```python
from build123d import *

# Parameters (mm, degrees)
BOSS_EXTRUDE1_DEPTH = 72
BOSS_EXTRUDE4_DEPTH = 6
SKETCH5_3_R         = 8.173204637
CUT_EXTRUDE1_DEPTH  = 6
BOSS_EXTRUDE6_START = 5
SKETCH7_R           = 15
BOSS_EXTRUDE6_DEPTH = 5
CUT_EXTRUDE3_START  = 5
SKETCH5_6_R         = 8.173204637
CUT_EXTRUDE3_DEPTH  = 5
RIB6_REACH          = 87.013
SKETCH18_WALL_W     = 218.674083686
SKETCH18_WALL_H     = 10
SKETCH20_R          = 6
CUT_EXTRUDE5_DEPTH  = 99.565967758
FILLET12_R          = 12


with BuildPart() as part:
    # Sketch2 → Boss-Extrude1 (new body)
    with BuildSketch(Plane(origin=(0, 0, 0), x_dir=(0, 0, -1), z_dir=(1, 0, 0))):
        Polygon((-17.5, 0), (-17.5, 6), (-12.5, 6), (-12.5, 10), (17.5, 10), (17.5, 0), align=None)
    extrude(amount=BOSS_EXTRUDE1_DEPTH)

    # Sketch5 → Boss-Extrude4 (add)
    with BuildSketch(Plane.XY.offset(12.5)):
        with BuildLine():
            Line((21, 60), (21, 20.340753373))
            ThreePointArc((21, 20.340753373), (17.971263459, 13.028736541), (10.659246627, 10))
            Line((10.659246627, 10), (61.340753373, 10))
            ThreePointArc((61.340753373, 10), (53.857333501, 15.45146146), (51, 24.258030049))
            Line((51, 24.258030049), (51, 60))
            ThreePointArc((51, 60), (36, 75), (21, 60))
        make_face()
    extrude(amount=-BOSS_EXTRUDE4_DEPTH)

    # Sketch5_3 → Cut-Extrude1 (cut)
    with BuildSketch(Plane.XY.offset(12.5)):
        with Locations((36, 60)):
            Circle(SKETCH5_3_R)
    extrude(amount=-CUT_EXTRUDE1_DEPTH, mode=Mode.SUBTRACT)

    # Sketch7 → Boss-Extrude6 (add)
    with BuildSketch(Plane.XY.offset(12.5).offset(BOSS_EXTRUDE6_START)):
        with Locations((36, 60)):
            Circle(SKETCH7_R)
    extrude(amount=-BOSS_EXTRUDE6_DEPTH)

    # Sketch5_6 → Cut-Extrude3 (cut)
    with BuildSketch(Plane.XY.offset(12.5).offset(CUT_EXTRUDE3_START)):
        with Locations((36, 60)):
            Circle(SKETCH5_6_R)
    extrude(amount=-CUT_EXTRUDE3_DEPTH, mode=Mode.SUBTRACT)

    # Sketch18 wall → Rib6 (add, up to next)
    with BuildSketch(Plane(origin=(36, 30, -5.5), x_dir=(0, -0.857492925713, -0.514495755428), z_dir=(0, 0.514495755428, -0.857492925713)), mode=Mode.PRIVATE) as rib6_sk1:
        Rectangle(SKETCH18_WALL_W, SKETCH18_WALL_H)
    rib6_tool1 = extrude(rib6_sk1.sketch, amount=-RIB6_REACH, mode=Mode.PRIVATE) - part.part
    add(rib6_tool1.solids().sort_by_distance((36, 30, -5.5))[0])

    # Sketch20 → Cut-Extrude5 (cut, through all)
    with BuildSketch(Plane(origin=(0, 10, 0), x_dir=(1, 0, 0), z_dir=(0, 1, 0))):
        with Locations(Location((12, 5.5, 0), (0, 0, 270))):
            Circle(SKETCH20_R)
        with Locations(Location((60, 5.5, 0), (0, 0, 270))):
            Circle(SKETCH20_R)
    extrude(amount=-CUT_EXTRUDE5_DEPTH, mode=Mode.SUBTRACT)

    # Fillet12
    fillet12_edges = [part.edges().sort_by_distance(p)[0] for p in [
        (0, 5, -17.5),
        (72, 5, -17.5),
    ]]
    fillet(fillet12_edges, radius=FILLET12_R)


solid = part.part
```
Part model, mm, in its own coordinate system. A direction names the side the tool comes from. Round coordinates to 2 decimals unless told otherwise and drop trailing zeros. Write each loop counter-clockwise with the first axis right and the second up, starting at its lowest first coordinate (ties: lowest second). Pieces come first, ordered by that corner, then holes. Notation, with made-up numbers: M -5,59 L 32,59 A11 ccw 32,75 Z; hole C 84.5,8.5 d7. An arc over 180 degrees is marked long. Answer as CSV lines item,"result". Start each with the question number.
1) Band-saw the part on B-B (z = 9). List the corners of the cut face in (x, y), then the cut area to 3 significant figures.
2) Mould opens along Z. For faces 4 (the face through (18.05, 13.11, 9.54)), 5 (the face through (6.143, 5.07, -6.801)), 6 (the face through (41.3, 35.7, 6.5)) say: +Z half, -Z half, draft (parallel to the pull), parting line (faces both ways), or undercut.
3) Band-saw the part on C-C (y = 26). List the corners of the cut face in (x, z).
4) Drop flat-ended pins along their axis: pin 1 (4 mm diameter, centred on y = 38, z = 6.5, fed in from +X); pin 2 (7 mm diameter, centred on x = 60, z = -5.5, fed in from -Y); pin 3 (1.5 mm diameter, centred on y = 22, z = 4.5, fed in from +X); pin 4 (12 mm diameter, centred on y = 22.5, z = -4.5, fed in from -X). Give the stop position or say it passes through.
5) Which spindle directions (+Z, -Z, +X, -X, +Y, -Y) get a long thin tool onto all of the face, cutting with end or side? Do faces 1 (the face through (34.047, 74.872, 13.299)), 2 (the face through (21, 40, 10)), 3 (the face through (19, 10, -2)). Say none if no direction does.
6) Drill centre lines: L1, parallel to X at y = 7, z = -5.5; L2, parallel to Y at x = 36, z = 15; L3, parallel to Z at x = 22, y = 62. Where is each one in solid material? Low to high.
7) Band-saw the part on A-A (x = 36). List the corners of the cut face in (y, z), then the cut area to 3 significant figures.
8) Band-saw the part on D-D (z = -6.5). List the corners of the cut face in (x, y).
Worked out:
1,outline,"M 0,0 L 72,0 L 72,10 L 61.34,10 A15 cw 51,24.26 L 51,60 A15 ccw 21,60 L 21,20.34 A10.34 cw 10.66,10 L 0,10 Z; hole C 36,60 d16.35"
1,area,"2,430 mm²"
2,face 4,"draft"
2,face 5,"undercut"
2,face 6,"-Z half"
3,outline,"M 21,6.5 L 31,6.5 L 31,-7.9 L 41,-7.9 L 41,6.5 L 51,6.5 L 51,12.5 L 21,12.5 Z"
4,pin 1,"x = 51"
4,pin 2,"through"
4,pin 3,"x = 41"
4,pin 4,"x = 31"
5,face 1,"+Z"
5,face 2,"+Z, -Z, -X, +Y"
5,face 3,"-Z, -X, +Y"
6,L1,"0 to 6, 18 to 54, 66 to 72"
6,L2,"0 to 6, 45 to 51.83, 68.17 to 75"
6,L3,"6.5 to 17.5"
7,outline,"M 0,-17.5 L 10,-17.5 L 50,6.5 L 51.83,6.5 L 51.83,17.5 L 45,17.5 L 45,12.5 L 6,12.5 L 6,17.5 L 0,17.5 Z; M 68.17,6.5 L 75,6.5 L 75,17.5 L 68.17,17.5 Z"
7,area,"1,170 mm²"
8,outline,"M 0.04,0 L 6.08,0 L 6.08,10 L 0.04,10 Z; M 17.92,0 L 54.08,0 L 54.08,10 L 41,10 L 41,28.33 L 31,28.33 L 31,10 L 17.92,10 Z; M 65.92,0 L 71.96,0 L 71.96,10 L 65.92,10 Z"
